Check sheet for the modelled part. Datum: model origin and axes. Units: mm. A direction names the side the tool comes from. Round coordinates to 2 decimals unless told otherwise and drop trailing zeros. Write each loop counter-clockwise with the first axis right and the second up, starting at its lowest first coordinate (ties: lowest second). Pieces come first, ordered by that corner, then holes.
Item 1: Section check A-A, the plane x = 0. State how many separate pieces and enclosed holes the cut face has, plus the area to 3 significant figures.
Item 2: Material ranges on line 1 along X through (y, z) = (37, -1); line 2 along X through (y, z) = (37.5, 3.5); line 3 along Z through (x, y) = (50.5, 76), recorded low to high.
Item 3: Release check for a two-part mould opening along Z. For faces 5 (the cylindrical face through (22.4, -7.1, 139.5)), 6 (the cylindrical face through (56.03, -36.33, -0.11)), 7 (the flat face through (-42.4, 21.9, 7.5)) record: pulls with the +Z half, pulls with the -Z half, needs draft (parallel to the pull), parting line crosses it, or undercut.
Item 4: Section check B-B, the plane z = 73. Record the cut outline in (x, y), plus the area to 3 significant figures.
Item 5: Section check C-C, the plane x = -66.5. Record the cut outline in (y, z), plus the area to 3 significant figures.
Item 6: Set-up check for faces 1 (the cylindrical face through (-56.967, -41.653, -0.105)), 2 (the cylindrical face through (23.846, -7.509, 143.055)), 3 (the flat face through (19.1, -10.4, 152.5)), 4 (the flat face through (40, 42, -7.5)): record each of +Z, -Z, +X, -X, +Y, -Y from which the full face is reachable in a straight line by a thin tool's end or side.
Item 7: Depth check by flat-ended pin: pin 1 (8 mm diameter, centred on x = -71, y = 28.5, fed in from +Z); pin 2 (3 mm diameter, centred on x = -32, y = 53, fed in from -Z); pin 3 (5 mm diameter, centred on y = 9.5, z = 125, fed in from -X). Enter the tip coordinate at first touch or a pass-through.
Autodesk Inventor part; units mm, degrees
ref_plane "YZ Plane" through (0, 0, 0) normal (1, 0, 0) x (0, 1, 0)
ref_plane "XZ Plane" through (0, 0, 0) normal (0, 1, 0) x (-1, 0, 0)
ref_plane "XY Plane" through (0, 0, 0) normal (0, 0, 1) x (1, 0, 0)
sketch "Sketch1" plane through (-207.0981, -171.1026, -7.5) normal (0, 0, 1) x (1, 0, 0)
  circle A0 centre (207.0981, 171.1026) radius 92.5
  dimension "d40" = 185
extrude "ExtrusionBlind1" add sketch "Sketch1" along normal blind 15
sketch "Sketch2" plane through (-207.0981, -171.1026, -7.5) normal (0, 0, 1) x (1, 0, 0)
  circle A0 centre (207.0981, 171.1026) radius 57.5
  circle A1 centre (207.0981, 171.1026) radius 92.5
  dimension "d41" = 115
extrude "ExtrusionBlind2" add sketch "Sketch2" against normal blind 10 contours A0
chamfer "Chamfer1" distance 2 angle 30 1 edges at (-57.5, 0, -17.5) measured on face at (-40.0277, -41.2799, -14.1667)
sketch "Sketch4" plane through (0, 0, 7.5) normal (0, 0, 1) x (1, 0, 0)
  circle A0 centre (0, 0) radius 32.5
  circle A1 centre (0, 0) radius 92.5
  dimension "d42" = 65
extrude "ExtrusionBlind3" add sketch "Sketch4" along normal blind 20 contours A0
fillet "Fillet1" radius 15 1 edges at (-32.5, 0, 7.5)
sketch "Sketch5" plane through (0, 0, 27.5) normal (0, 0, 1) x (1, 0, 0)
  circle A0 centre (0, 0) radius 25
  circle A1 centre (0, 0) radius 32.5
  dimension "d43" = 50
extrude "ExtrusionBlind4" add sketch "Sketch5" along normal blind 110 contours A0
sketch "Sketch6" plane through (0, 0, 137.5) normal (0, 0, 1) x (1, 0, 0)
  circle A0 centre (0, 0) radius 23.5
  circle A1 centre (0, 0) radius 25
  dimension "d44" = 47
extrude "ExtrusionBlind5" add sketch "Sketch6" along normal blind 4.15 contours A0
sketch "Sketch7" plane through (0, 0, 141.65) normal (0, 0, 1) x (1, 0, 0)
  circle A0 centre (0, 0) radius 25
  circle A1 centre (0, 0) radius 23.5
  dimension "d45" = 50
extrude "ExtrusionBlind6" add sketch "Sketch7" along normal blind 4.85 contours A0 | A1
chamfer "Chamfer2" distance 2 angle 30 1 edges at (-25, 0, 146.5) measured on face at (24.9189, -2.0117, 144.8833)
sketch "Sketch8" plane through (0, 0, 146.5) normal (0, 0, 1) x (1, 0, 0)
  circle A0 centre (0, 0) radius 21.5
  circle A1 centre (0, 0) radius 23.8453
  dimension "d46" = 43
extrude "ExtrusionBlind7" add sketch "Sketch8" along normal blind 6 contours A0
sketch "Sketch9" plane through (0, 0, 152.5) normal (0, 0, 1) x (1, 0, 0)
  circle A0 centre (0, 0) radius 23.6
  circle A1 centre (0, 0) radius 21.5
  dimension "d47" = 47.2
extrude "ExtrusionBlind8" add sketch "Sketch9" along normal blind 26 contours A0 | A1
chamfer "Chamfer3" distance 2 angle 45 1 edges at (-23.6, 0, 178.5)
sketch "Sketch12" plane through (0, 0, 7.5) normal (0, 0, 1) x (1, 0, 0)
  circle A0 centre (0, 0) radius 92.5
  line L0 (0, 0) -> (0, 75) construction
  dimension "d51" = 75
hole "Hole2" at (0, 75, 7.5) direction (0, 0, -1) diameter 18 end through all
pattern_circular "Circular Pattern2" count 6 over 360 about axis through (0, 0, -7.5) along (0, 0, 1) of "Hole2"
properties part number "7055-191 PART1" material "Steel, Mild"
Values found:
1. separate pieces: 3
1. enclosed holes: 0
1. area: 12,200 mm2
2. line 1: x = -84.78 to -73.94, -55.97 to 55.97, 73.94 to 84.78
2. line 2: x = -84.56 to -73.95, -55.95 to 55.95, 73.95 to 84.56
2. line 3: z = -7.5 to 7.5
3. face 5: undercut
3. face 6: needs draft
3. face 7: pulls with the +Z half
4. outline: circle Ø50 at (0, 0)
4. area: 1,960 mm2
5. outline: (-64.3, -7.5) - (-46.37, -7.5) - (-46.37, 7.5) - (-64.3, 7.5) - close; (-28.63, -7.5) - (28.63, -7.5) - (28.63, 7.5) - (-28.63, 7.5) - close; (46.37, -7.5) - (64.3, -7.5) - (64.3, 7.5) - (46.37, 7.5) - close
5. area: 1,400 mm2
6. face 1: +Z, -Z
6. face 2: +Z
6. face 3: none
6. face 4: -Z
7. pin 1: stops at z = 7.5
7. pin 2: stops at z = -7.5
7. pin 3: stops at x = -24
